Work out the finished part from the listing and answer in its coordinate system (mm). Round coordinates to 2 decimals unless told otherwise and drop trailing zeros. Order: outer loops, then holes, each group sorted by start corner. A loop starts at its lowest first (then second) coordinate and runs counter-clockwise, first axis right, second up. Notation, with made-up numbers: (38, 27) - (66, 27) arc R11 cw to (66, 35) - close; hole circle Ø3 at (77, -40). An arc over 180 degrees is marked (long way). Answer in a Markdown table with one row per item.
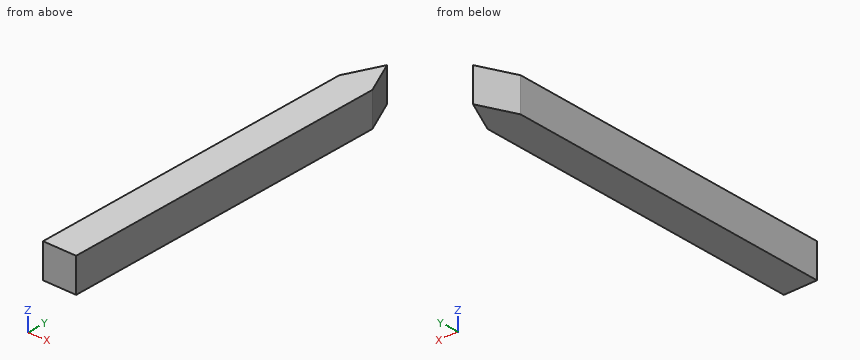
from build123d import *

# Parameters (mm, degrees)
F0_W     = 55
F0_H     = 555
F1_DEPTH = 56


with BuildPart() as f1:
    # F0 (on Top) → F1 (new body)
    with BuildSketch(Plane.XY):
        with Locations((-27.5, 277.5)):
            Rectangle(F0_W, F0_H)
        Polygon((-55, 555), (0, 555), (-27.5, 613.364637), align=None)
    extrude(amount=F1_DEPTH)


solid = f1.part
1) Find section A-A, the plane z = 16. Give the vertices of the cut face in (x, y), then the cut area to 3 significant figures.
Filled in:
| item | result |
|---|---|
| outline | (-55, 0) - (0, 0) - (0, 555) - (-27.5, 613.36) - (-55, 555) - close |
| area | 32,100 mm^2 |
2) This flat-tipped pin is pushed along its axis until it touches: pin 1 (1.5 mm diameter, centred on x = -14.5, z = 20, fed in from +Y). Where does it stop, or does it pass through?
Filled in:
| item | result |
|---|---|
| pin 1 | stops at y = 587.37 |
3) Find the intervals of material crossed by probe 1 along Y at (x, z) = (-30, 38); probe 2 along Y at (x, z) = (-20.5, 5.5), in increasing order. Write a range as from..to.
Filled in:
| item | result |
|---|---|
| probe 1 | y = 0..608.06 |
| probe 2 | y = 0..598.51 |
4) Find section C-C, the plane y = 570. Give the vertices of the cut face in (x, z), then the cut area to 3 significant figures.
Filled in:
| item | result |
|---|---|
| outline | (-47.93, 0) - (-7.07, 0) - (-7.07, 56) - (-47.93, 56) - close |
| area | 2,290 mm^2 |
5) Find section B-B, the plane x = -9. Give the vertices of the cut face in (y, z).
Filled in:
| item | result |
|---|---|
| outline | (0, 0) - (574.1, 0) - (574.1, 56) - (0, 56) - close |
